from build123d import *

# Parameters (mm, degrees)
SKETCH_1_R      = 1.5
SKETCH_1_R_2    = 5
EXTRUDE_1_DEPTH = 3.5
SKETCH_1_2_R    = 1.5
SKETCH_1_2_R_2  = 5
EXTRUDE_2_DEPTH = 6.5
FILLET_3_R      = 10
FILLET_4_R      = 10
FILLET_5_R      = 30


with BuildPart() as part:
    # Sketch 1 → Extrude 1 (new body)
    with BuildSketch(Plane(origin=(0, 0, 0), x_dir=(1, 0, 0), z_dir=(0, 1, 0))):
        with BuildLine():
            Line((0, 0), (53, 0))
            Line((53, 0), (53, 20))
            Line((53, 20), (46.5, 20))
            ThreePointArc((46.5, 20), (33.418524548, 25.418524548), (28, 38.5))
            ThreePointArc((28, 38.5), (14, 52.5), (0, 38.5))
            Line((0, 38.5), (0, 0))
        make_face()
        with Locations(Location((14, 44.5, 0), (0, 0, 270))):
            Circle(SKETCH_1_R, mode=Mode.SUBTRACT)
        with Locations(Location((19.196152423, 35.5, 0), (0, 0, 270))):
            Circle(SKETCH_1_R, mode=Mode.SUBTRACT)
        with Locations(Location((43, 10, 0), (0, 0, 270))):
            Circle(SKETCH_1_R, mode=Mode.SUBTRACT)
        with Locations(Location((14, 26, 0), (0, 0, 270))):
            Circle(SKETCH_1_R_2, mode=Mode.SUBTRACT)
        with Locations(Location((8.803847577, 35.5, 0), (0, 0, 270))):
            Circle(SKETCH_1_R, mode=Mode.SUBTRACT)
        with Locations(Location((25.441221962, 17.093145751, 0), (0, 0, 270))):
            Circle(SKETCH_1_R, mode=Mode.SUBTRACT)
    extrude(amount=EXTRUDE_1_DEPTH)

    # Sketch 1_2 → Extrude 2 (add)
    with BuildSketch(Plane(origin=(0, 0, 0), x_dir=(1, 0, 0), z_dir=(0, 1, 0))):
        with BuildLine():
            Line((0, 0), (53, 0))
            Line((53, 0), (53, 20))
            Line((53, 20), (46.5, 20))
            ThreePointArc((46.5, 20), (33.418524548, 25.418524548), (28, 38.5))
            ThreePointArc((28, 38.5), (14, 52.5), (0, 38.5))
            Line((0, 38.5), (0, 0))
        make_face()
        with Locations(Location((14, 44.5, 0), (0, 0, 270))):
            Circle(SKETCH_1_2_R, mode=Mode.SUBTRACT)
        with Locations(Location((19.196152423, 35.5, 0), (0, 0, 270))):
            Circle(SKETCH_1_2_R, mode=Mode.SUBTRACT)
        with Locations(Location((43, 10, 0), (0, 0, 270))):
            Circle(SKETCH_1_2_R, mode=Mode.SUBTRACT)
        with Locations(Location((14, 26, 0), (0, 0, 270))):
            Circle(SKETCH_1_2_R_2, mode=Mode.SUBTRACT)
        with Locations(Location((8.803847577, 35.5, 0), (0, 0, 270))):
            Circle(SKETCH_1_2_R, mode=Mode.SUBTRACT)
        with Locations(Location((25.441221962, 17.093145751, 0), (0, 0, 270))):
            Circle(SKETCH_1_2_R, mode=Mode.SUBTRACT)
    extrude(amount=EXTRUDE_2_DEPTH)

    # Fillet 3
    fillet_3_edges = [part.edges().sort_by_distance(p)[0] for p in [
        (53, 3.25, 0),
    ]]
    fillet(fillet_3_edges, radius=FILLET_3_R)

    # Fillet 4
    fillet_4_edges = [part.edges().sort_by_distance(p)[0] for p in [
        (53, 3.25, -20),
    ]]
    fillet(fillet_4_edges, radius=FILLET_4_R)

    # Fillet 5
    fillet_5_edges = [part.edges().sort_by_distance(p)[0] for p in [
        (0, 3.25, 0),
    ]]
    fillet(fillet_5_edges, radius=FILLET_5_R)


solid = part.part
Design review of the part built by this model. Coordinates are the model's own, in mm. Give positions to 0.01 mm unless a question says otherwise; leave off trailing zeros. Loops run counter-clockwise (first coordinate to the right, second up) from the corner with the lowest first, then second, coordinate; pieces in that order, holes last. Notation, with made-up numbers: (56, 59.5) - (105, 59.5) arc R17 cw to (105, 71.5) - close; hole circle Ø9 at (-3.5, 16.25). An arc over 180 degrees is marked (long way). Write item = value, one per line.
1) Take a section at B-B on z = -35.5. State the section outline as (x, y) points, and give its area (3 significant figures).
Result sheet:
outline = (0, 0) - (7.3, 0) - (7.3, 6.5) - (0, 6.5) - close; (10.3, 0) - (17.7, 0) - (17.7, 6.5) - (10.3, 6.5) - close; (20.7, 0) - (28.24, 0) - (28.24, 6.5) - (20.7, 6.5) - close
area = 145 mm2
2) Draft analysis for pull direction Z (two halves, no side actions). For faces 1 (the face through (14, 3, -46)), 2 (the face through (36, 3, 0)), 3 (the face through (20, 0, -21)), state which applies: +Z half, -Z half, draft (parallel to the pull), parting line (faces both ways), or undercut.
Result sheet:
face_1 = undercut
face_2 = +Z half
face_3 = draft
3) Clearance check with a flat-ended pin moving along its axis: pin 1 Ø1 at (x, y) = (22.5, 3) entering from +Z. State where the tip first meets the part, or that it passes through.
Result sheet:
pin_1 = -0.83
4) Take a section at D-D on z = -44.5. State the section outline as (x, y) points.
Result sheet:
outline = (1.35, 0) - (12.5, 0) - (12.5, 6.5) - (1.35, 6.5) - close; (15.5, 0) - (26.65, 0) - (26.65, 6.5) - (15.5, 6.5) - close
5) To check wall thickness, follow line 1 (X direction, y = 2.75, z = -35.5); line 2 (Z direction, x = 18, y = 4.75); line 3 (Z direction, x = 16.5, y = 1). State the ranges of each line that lie inside material, in increasing order.
Result sheet:
line_1 = 0 to 7.3, 10.3 to 17.7, 20.7 to 28.24
line_2 = -51.92 to -36.41, -34.59 to -29, -23 to -2.5
line_3 = -52.27 to -30.33, -21.67 to -3.21
6) Take a section at A-A on z = -25. State the section outline as (x, y) points, and give its area (3 significant figures).
Result sheet:
outline = (0.42, 0) - (9.1, 0) - (9.1, 6.5) - (0.42, 6.5) - close; (18.9, 0) - (33.85, 0) - (33.85, 6.5) - (18.9, 6.5) - close
area = 154 mm2
7) Take a section at C-C on y = 1. Count the separate pieces of the cut face and the enclosed holes in it, and give its area (3 significant figures).
Result sheet:
separate_pieces = 1
enclosed_holes = 6
area = 1,610 mm2
